from build123d import *

# Parameters (mm, degrees)
SKETCH_W        = 97.5
SKETCH_H        = 13
PAD_DEPTH       = 8
SKETCH001_R     = 1.7
POCKET_DEPTH    = 20
SKETCH002_W     = 8
SKETCH002_H     = 5
POCKET001_DEPTH = 20
FILLET_R        = 3


with BuildPart() as part:
    # Sketch → Pad (new body)
    with BuildSketch(Plane.XY):
        with Locations((1.25, 0)):
            Rectangle(SKETCH_W, SKETCH_H)
    extrude(amount=PAD_DEPTH)

    # Sketch001 (on Face1 of Pad) → Pocket (cut)
    with BuildSketch(Plane.XZ.offset(6.5)):
        with Locations((-44.5, 4)):
            Circle(SKETCH001_R)
        with Locations((47, 4)):
            Circle(SKETCH001_R)
    extrude(amount=-POCKET_DEPTH, mode=Mode.SUBTRACT)

    # Sketch002 (on Face4 of Pocket) → Pocket001 (cut)
    with BuildSketch(Plane.XY.offset(8)):
        with Locations((-43.5, 0)):
            Rectangle(SKETCH002_W, SKETCH002_H)
        with Locations((46, 0)):
            Rectangle(SKETCH002_W, SKETCH002_H)
    extrude(amount=-POCKET001_DEPTH, mode=Mode.SUBTRACT)

    # Fillet
    fillet_edges = [part.edges().sort_by_distance(p)[0] for p in [
        (50, 4.5, 8),
        (50, -4.5, 8),
        (50, -4.5, 0),
        (50, 4.5, 0),
        (-47.5, -4.5, 8),
        (-47.5, -4.5, 0),
        (-47.5, 4.5, 0),
        (-47.5, 4.5, 8),
    ]]
    fillet(fillet_edges, radius=FILLET_R)


solid = part.part
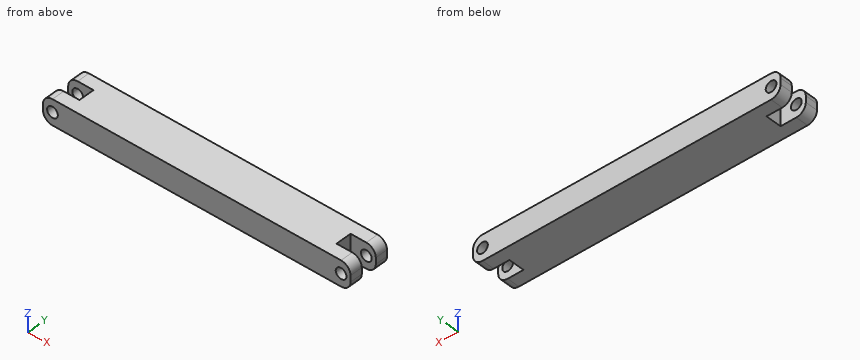
Source: CAD feature listing. Evaluate the final solid. Frame: model axes, mm. Give positions to 0.01 mm unless a question says otherwise; leave off trailing zeros. Write each loop counter-clockwise with the first axis right and the second up, starting at its lowest first coordinate (ties: lowest second). Pieces come first, ordered by that corner, then holes. Notation, with made-up numbers: M 5,66 L 60,66 A14 ccw 60,88 Z; hole C 45,6.25 d5. An arc over 180 degrees is marked long. Return JSON: item names as keys, results as strings. Group by question number.
1) Cut plane C-C, the plane y = 0.5. Output: boundary loops of the cut face in (x, z).
2) Cut plane B-B, the plane y = 4.5. Output: boundary loops of the cut face in (x, z), then the cut area to 3 significant figures.
3) Cut plane A-A, the plane z = 4. Output: boundary loops of the cut face in (x, y).
4) Ray query, L1, parallel to Z at x = 47, y = 4.15; L2, parallel to Y at x = -42, z = 4.5; L3, parallel to X at y = -3.5, z = 3. Return the intervals inside material, ascending.
5) First-contact query: pin 1 Ø4 at (y, z) = (0, 3) entering from +X; pin 2 Ø1.5 at (y, z) = (0.5, 5.5) entering from -X; pin 3 Ø5 at (x, y) = (39, -2) entering from -Z; pin 4 Ø2 at (y, z) = (2, 6) entering from -X. Flat tips, straight axial feed; report the tip coordinate or a pass-through.
Data:
{
 "1": {"outline": "M -39.5,0 L 42,0 L 42,8 L -39.5,8 Z"},
 "2": {"outline": "M -47.5,3 A3 ccw -44.5,0 L 47,0 A3 ccw 50,3 L 50,5 A3 ccw 47,8 L -44.5,8 A3 ccw -47.5,5 Z; hole C -44.5,4 d3.4; hole C 47,4 d3.4", "area": "754 mm²"},
 "3": {"outline": "M -47.5,-6.5 L -46.2,-6.5 L -46.2,-2.5 L -47.5,-2.5 Z; M -47.5,2.5 L -46.2,2.5 L -46.2,6.5 L -47.5,6.5 Z; M -42.8,-6.5 L 45.3,-6.5 L 45.3,-2.5 L 42,-2.5 L 42,2.5 L 45.3,2.5 L 45.3,6.5 L -42.8,6.5 L -42.8,2.5 L -39.5,2.5 L -39.5,-2.5 L -42.8,-2.5 Z; M 48.7,-6.5 L 50,-6.5 L 50,-2.5 L 48.7,-2.5 Z; M 48.7,2.5 L 50,2.5 L 50,6.5 L 48.7,6.5 Z"},
 "4": {"L1": "z = 0 to 2.3, 5.7 to 8", "L2": "y = -6.5 to -2.5, 2.5 to 6.5", "L3": "x = -47.5 to -45.87, -43.13 to 45.63, 48.37 to 50"},
 "5": {"pin 1": "stops at x = 42", "pin 2": "stops at x = -39.5", "pin 3": "stops at z = 0", "pin 4": "stops at x = -47.5"}
}
